The listing builds one solid part. Answer for the finished solid, in the listing's coordinates (mm). A direction names the side the tool comes from. Round coordinates to 2 decimals unless told otherwise and drop trailing zeros. Write each loop counter-clockwise with the first axis right and the second up, starting at its lowest first coordinate (ties: lowest second). Pieces come first, ordered by that corner, then holes.
Item 1: Find section C-C on y = 0. Give the vertices of the cut face in (x, z).
Item 2: Find the intervals of material crossed by probe 1 along Y at (x, z) = (0, -24.75); probe 2 along Y at (x, z) = (-4, 0); probe 3 along X at (y, z) = (1.25, -13.5), in increasing order.
Item 3: Find section A-A on x = 0. Give the vertices of the cut face in (y, z), then the cut area to 3 significant figures.
Item 4: A tool of negligible diameter and unlimited length cuts with its end or side. For faces 1 (the face through (0, -6, -33)), 2 (the face through (8.545, -3.543, -20.681)), 3 (the face through (-0.08, -9.25, -7.23)), from which of +Z, -Z, +X, -X, +Y, -Y can it reach the whole face along a straight path? Write none if from no direction.
Item 5: Find section D-D on z = -27. Give the vertices of the cut face in (x, y), then the cut area to 3 significant figures.
Item 6: Find section B-B on z = 0. Give the vertices of the cut face in (x, y).
Item 7: For a pull along Y with two mould halves and no side action, classify faces 4 (the face through (-25, 11.2, 1)), 5 (the face through (-2.185, -3.815, 12.114)), 6 (the face through (-5.714, 0.251, -20.325)) as +Y half, -Y half, draft (parallel to the pull), parting line (faces both ways), or undercut.
Item 8: Each of these flat-tipped pins is pushed along its axis until it touches: pin 1 (2 mm diameter, centred on x = -11, z = -27.5, fed in from -Y); pin 2 (5 mm diameter, centred on x = -3, z = 3, fed in from -Y); pin 3 (6 mm diameter, centred on y = 9.5, z = -10.5, fed in from +X). Where does it stop, or does it pass through?
```python
from build123d import *

# Parameters (mm, degrees)
SKIZZE3_R                       = 9.25
SCHNITT_LINEAR_AUSTRAGEN1_DEPTH = 30
SKIZZE5_R                       = 9.25
SKIZZE5_R_2                     = 5.72
AUFSATZ_LINEAR_AUSTRAGEN1_DEPTH = 25


with BuildPart() as part:
    # Skizze1 → Rotation1 (revolve)
    with BuildSketch(Plane.XY, mode=Mode.PRIVATE) as rotation1_sk:
        with BuildLine():
            Line((-25, 12.7), (20, 12.7))
            ThreePointArc((20, 12.7), (23.535533906, 11.235533906), (25, 7.7))
            Line((25, 7.7), (25, 0))
            Line((25, 0), (23.01981108, 0))
            Line((23.01981108, 0), (23.01981108, 6.05))
            ThreePointArc((23.01981108, 6.05), (21.555344986, 9.585533906), (18.01981108, 11.05))
            Line((18.01981108, 11.05), (-25, 11.05))
            Line((-25, 11.05), (-25, 12.7))
        make_face()
    revolve(rotation1_sk.sketch.rotate(Axis((-16.35087822, 0, 0), (1, 0, 0)), 90), axis=Axis((-16.35087822, 0, 0), (1, 0, 0)))

    # Skizze2 → Schnitt-Rotation1 (revolve, cut)
    with BuildSketch(Plane(origin=(0, 0, 0), x_dir=(1, 0, 0), z_dir=(0, 1, 0)), mode=Mode.PRIVATE) as schnitt_rotation1_sk:
        Polygon((22, 0), (22, 8), (25, 9), (25, 0), align=None)
    revolve(schnitt_rotation1_sk.sketch.rotate(Axis((-29.523851761, 0, 0), (1, 0, 0)), 180), axis=Axis((-29.523851761, 0, 0), (1, 0, 0)), mode=Mode.SUBTRACT)

    # Skizze3 → Schnitt-Linear austragen1 (cut)
    with BuildSketch(Plane.XY):
        Circle(SKIZZE3_R)
    extrude(amount=-SCHNITT_LINEAR_AUSTRAGEN1_DEPTH, mode=Mode.SUBTRACT)

    # Skizze5 → Aufsatz-Linear austragen1 (add)
    with BuildSketch(Plane.XY.offset(-8)):
        Circle(SKIZZE5_R)
        Circle(SKIZZE5_R_2, mode=Mode.SUBTRACT)
    extrude(amount=-AUFSATZ_LINEAR_AUSTRAGEN1_DEPTH)


solid = part.part
```
Check values:
1. outline: (-25, -12.7) - (-9.25, -12.7) - (-9.25, -33) - (-5.72, -33) - (-5.72, -8) - (-9.25, -8) - (-9.25, -11.05) - (-25, -11.05) - close; (-25, 11.05) - (18.02, 11.05) arc R5 cw to (22.54, 8.18) - (24.84, 8.95) arc R5 ccw to (20, 12.7) - (-25, 12.7) - close; (5.72, -33) - (9.25, -33) - (9.25, -12.7) - (20, -12.7) arc R5 ccw to (24.84, -8.95) - (22.54, -8.18) arc R5 cw to (18.02, -11.05) - (9.25, -11.05) - (9.25, -8) - (5.72, -8) - close
2. probe 1: y = -9.25 to -5.72, 5.72 to 9.25
2. probe 2: y = -12.7 to -11.05, 11.05 to 12.7
2. probe 3: x = -9.17 to -5.58, 5.58 to 9.17
3. outline: (-9.25, -33) - (-5.72, -33) - (-5.72, -8) - (-9.25, -8) - (-9.25, -6.04) arc R11.05 cw (long way) to (9.25, -6.04) - (9.25, -8) - (5.72, -8) - (5.72, -33) - (9.25, -33) - (9.25, -8.7) arc R12.7 ccw (long way) to (-9.25, -8.7) - close
3. area: 265 mm2
4. face 1: -Z, +X, -X, +Y, -Y
4. face 2: -Z
4. face 3: none
5. outline: circle Ø18.5 at (0, 0); hole circle Ø11.44 at (0, 0)
5. area: 166 mm2
6. outline: (-25, -12.7) - (20, -12.7) arc R5 ccw to (24.84, -8.95) - (22.54, -8.18) arc R5 cw to (18.02, -11.05) - (-25, -11.05) - close; (-25, 11.05) - (18.02, 11.05) arc R5 cw to (22.54, 8.18) - (24.84, 8.95) arc R5 ccw to (20, 12.7) - (-25, 12.7) - close
7. face 4: draft
7. face 5: parting line
7. face 6: undercut
8. pin 1: passes through
8. pin 2: stops at y = -12.69
8. pin 3: stops at x = 23.61
